```python
from build123d import *

# Parameters (mm, degrees)
F0_R     = 2.5
F0_R_2   = 1.4
F1_DEPTH = 6
F2_DEPTH = 3.5
F3_DEPTH = 2


with BuildPart() as f1:
    # F0 (on Top) → F1 (new body)
    with BuildSketch(Plane.XY):
        Circle(F0_R)
        Circle(F0_R_2, mode=Mode.SUBTRACT)
    extrude(amount=F1_DEPTH)

    # F0 (on Top) → F2 (join)
    with BuildSketch(Plane.XY):
        with BuildLine():
            ThreePointArc((3.9993347498, -0.0729490169), (3.999833684, -0.0364760251), (4, 0))
            ThreePointArc((4, 0), (3.999833684, 0.0364760251), (3.9993347498, 0.0729490169))
            Line((3.9993347498, 0.0729490169), (2.0628430767, 3.4270509831))
            ThreePointArc((2.0628430767, 3.4270509831), (2, 3.4641016151), (1.9364916731, 3.5))
            Line((1.9364916731, 3.5), (-1.9364916731, 3.5))
            ThreePointArc((-1.9364916731, 3.5), (-2, 3.4641016151), (-2.0628430767, 3.4270509831))
            Line((-2.0628430767, 3.4270509831), (-3.9993347498, 0.0729490169))
            ThreePointArc((-3.9993347498, 0.0729490169), (-4, 0), (-3.9993347498, -0.0729490169))
            Line((-3.9993347498, -0.0729490169), (-2.0628430767, -3.4270509831))
            ThreePointArc((-2.0628430767, -3.4270509831), (-2, -3.4641016151), (-1.9364916731, -3.5))
            Line((-1.9364916731, -3.5), (1.9364916731, -3.5))
            ThreePointArc((1.9364916731, -3.5), (2, -3.4641016151), (2.0628430767, -3.4270509831))
            Line((2.0628430767, -3.4270509831), (3.9993347498, -0.0729490169))
        make_face()
        Circle(F0_R, mode=Mode.SUBTRACT)
        with BuildLine():
            Line((-1.9364916731, 3.5), (1.9364916731, 3.5))
            ThreePointArc((1.9364916731, 3.5), (0, 4), (-1.9364916731, 3.5))
        make_face()
        with BuildLine():
            Line((-3.9993347498, 0.0729490169), (-2.0628430767, 3.4270509831))
            ThreePointArc((-2.0628430767, 3.4270509831), (-3.4641016151, 2), (-3.9993347498, 0.0729490169))
        make_face()
        with BuildLine():
            ThreePointArc((-3.9993347498, -0.0729490169), (-3.4641016151, -2), (-2.0628430767, -3.4270509831))
            Line((-2.0628430767, -3.4270509831), (-3.9993347498, -0.0729490169))
        make_face()
        with BuildLine():
            ThreePointArc((-1.9364916731, -3.5), (0, -4), (1.9364916731, -3.5))
            Line((1.9364916731, -3.5), (-1.9364916731, -3.5))
        make_face()
        with BuildLine():
            ThreePointArc((2.0628430767, -3.4270509831), (3.4641016151, -2), (3.9993347498, -0.0729490169))
            Line((3.9993347498, -0.0729490169), (2.0628430767, -3.4270509831))
        make_face()
        with BuildLine():
            Line((2.0628430767, 3.4270509831), (3.9993347498, 0.0729490169))
            ThreePointArc((3.9993347498, 0.0729490169), (3.4641016151, 2), (2.0628430767, 3.4270509831))
        make_face()
    extrude(amount=F2_DEPTH)

    # F0 (on Top) → F3 (cut)
    with BuildSketch(Plane.XY):
        with BuildLine():
            ThreePointArc((3.9993347498, -0.0729490169), (3.999833684, -0.0364760251), (4, 0))
            ThreePointArc((4, 0), (3.999833684, 0.0364760251), (3.9993347498, 0.0729490169))
            Line((3.9993347498, 0.0729490169), (2.0628430767, 3.4270509831))
            ThreePointArc((2.0628430767, 3.4270509831), (2, 3.4641016151), (1.9364916731, 3.5))
            Line((1.9364916731, 3.5), (-1.9364916731, 3.5))
            ThreePointArc((-1.9364916731, 3.5), (-2, 3.4641016151), (-2.0628430767, 3.4270509831))
            Line((-2.0628430767, 3.4270509831), (-3.9993347498, 0.0729490169))
            ThreePointArc((-3.9993347498, 0.0729490169), (-4, 0), (-3.9993347498, -0.0729490169))
            Line((-3.9993347498, -0.0729490169), (-2.0628430767, -3.4270509831))
            ThreePointArc((-2.0628430767, -3.4270509831), (-2, -3.4641016151), (-1.9364916731, -3.5))
            Line((-1.9364916731, -3.5), (1.9364916731, -3.5))
            ThreePointArc((1.9364916731, -3.5), (2, -3.4641016151), (2.0628430767, -3.4270509831))
            Line((2.0628430767, -3.4270509831), (3.9993347498, -0.0729490169))
        make_face()
        Circle(F0_R, mode=Mode.SUBTRACT)
        Circle(F0_R)
        Circle(F0_R_2, mode=Mode.SUBTRACT)
    extrude(amount=F3_DEPTH, mode=Mode.SUBTRACT)


solid = f1.part
```
Part model, mm, in its own coordinate system. A direction names the side the tool comes from. Round coordinates to 2 decimals unless told otherwise and drop trailing zeros. Write each loop counter-clockwise with the first axis right and the second up, starting at its lowest first coordinate (ties: lowest second). Pieces come first, ordered by that corner, then holes. Notation, with made-up numbers: (77, -8.5) -> (125, -8.5) arc R24 cw to (125, 1.5) -> close; hole circle Ø4 at (21.25, 5). An arc over 180 degrees is marked (long way). Return JSON: item names as keys, results as strings. Group by question number.
Q1. Saw through at B-B on z = 0.8. Write the cut outline in (x, y), plus the area to 3 significant figures.
Q2. Mould opens along Y. For faces 4 (the flat face through (0, -3.5, 1)), 5 (the flat face through (-3.2, 1.8, 0)), 6 (the cylindrical face through (-0.54, -2.44, 4.73)), 7 (the flat face through (0, 3.5, 1)) say: pulls with the +Y half, pulls with the -Y half, needs draft (parallel to the pull), parting line crosses it, or undercut.
Q3. Which spindle directions (+Z, -Z, +X, -X, +Y, -Y) get a long thin tool onto all of the face, cutting with end or side? Do faces 1 (the flat face through (3, -1.8, 1)), 2 (the flat face through (1.1, -1.1, 6)), 3 (the flat face through (-2, -2, 3.5)). Say none if no direction does.
Q4. Probe L1, parallel to Y at x = 0, z = 5; L2, parallel to Z at x = -1.25, y = -1; L3, parallel to Z at x = 3.5, y = 0. List the from-to ranges inside material, lowest first. Write a range as [from, to].
Q5. Pin check, flat tips, straight feed: pin 1 (3 mm diameter, centred on x = -1, y = -1, fed in from -Z); pin 2 (3 mm diameter, centred on y = -2, z = 1, fed in from -X); pin 3 (0.6 mm diameter, centred on x = -1, z = 1, fed in from -Y). Stop position of each tip, or through.
Q6. Saw through at D-D on z = 3. Write the cut outline in (x, y).
Q7. Saw through at A-A on x = 0. Write the cut outline in (y, z), plus the area to 3 significant figures.
Q8. Saw through at C-C on y = -0.5. Write the cut outline in (x, z), plus the area to 3 significant figures.
Answer:
{
 "1": {"outline": "(-4, -0.07) arc R4 ccw to (-2.06, -3.43) -> close; (-4, 0.07) -> (-2.06, 3.43) arc R4 ccw to start; (-1.94, -3.5) arc R4 ccw to (1.94, -3.5) -> close; (-1.94, 3.5) -> (1.94, 3.5) arc R4 ccw to start; (2.06, -3.43) arc R4 ccw to (4, -0.07) -> close; (2.06, 3.43) -> (4, 0.07) arc R4 ccw to start", "area": "7.85 mm2"},
 "2": {"face 4": "undercut", "face 5": "needs draft", "face 6": "parting line crosses it", "face 7": "undercut"},
 "3": {"face 1": "-Z", "face 2": "+Z, +X, -X, +Y, -Y", "face 3": "+Z"},
 "4": {"L1": "[-2.5, -1.4], [1.4, 2.5]", "L2": "[2, 6]", "L3": "[2, 3.5]"},
 "5": {"pin 1": "z = 2", "pin 2": "x = -3.97", "pin 3": "y = -3.94"},
 "6": {"outline": "circle Ø8 at (0, 0); hole circle Ø2.8 at (0, 0)"},
 "7": {"outline": "(-4, 0) -> (-3.5, 0) -> (-3.5, 2) -> (-1.4, 2) -> (-1.4, 6) -> (-2.5, 6) -> (-2.5, 3.5) -> (-4, 3.5) -> close; (1.4, 2) -> (3.5, 2) -> (3.5, 0) -> (4, 0) -> (4, 3.5) -> (2.5, 3.5) -> (2.5, 6) -> (1.4, 6) -> close", "area": "15.3 mm2"},
 "8": {"outline": "(-3.97, 0) -> (-3.75, 0) -> (-3.75, 2) -> (-1.31, 2) -> (-1.31, 6) -> (-2.45, 6) -> (-2.45, 3.5) -> (-3.97, 3.5) -> close; (1.31, 2) -> (3.75, 2) -> (3.75, 0) -> (3.97, 0) -> (3.97, 3.5) -> (2.45, 3.5) -> (2.45, 6) -> (1.31, 6) -> close", "area": "14.6 mm2"}
}
